Can you work these out from the drawing? Everything is in mm from the part's minimum corner. A direction names the side the tool comes from. Coordinates: 2 decimals unless noted, no trailing zeros. Loops run counter-clockwise (first coordinate to the right, second up) from the corner with the lowest first, then second, coordinate; pieces in that order, holes last.
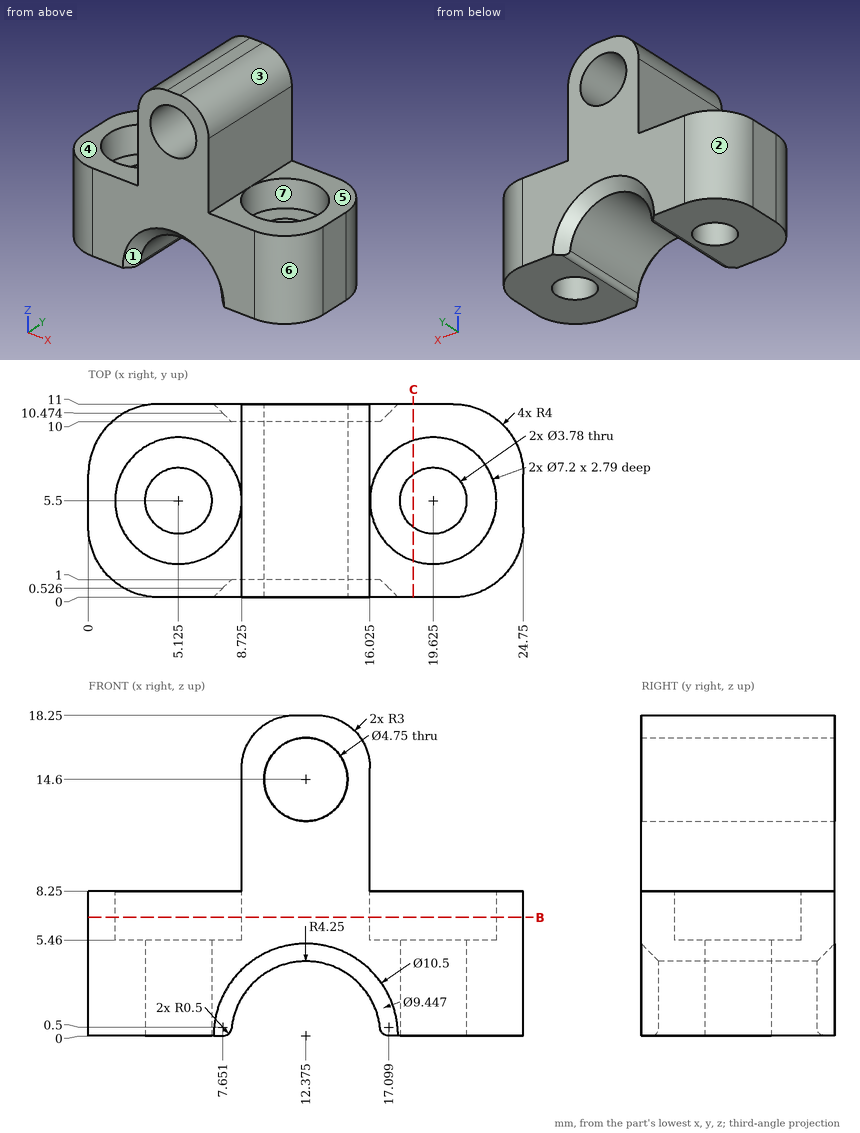
1. On a 3-axis mill with a long thin cutter (end or side, diameter ignored), from which of +Z, -Z, +X, -X, +Y, -Y can I reach the whole of each face in a straight line? I mean the marked faces 5, 6 and 7. Say none if no direction works.
2. We'd pull the mould along X, two halves only. Please class the marked faces 1, 2, 3 and 4: +X half, -X half, draft (parallel to the pull), parting line (faces both ways), or undercut.
3. For pin 1 (6 mm diameter, centred on x = 19.625, y = 5.5, fed in from +Z); pin 2 (1 mm diameter, centred on y = 5.5, z = 9, fed in from +X) (3 decimals); pin 3 (2 mm diameter, centred on y = 7, z = 10.5, fed in from -X) (3 decimals), each with a flat end and sliding along its axis, tell me the tip position at first contact or that it passes through.
4. I want a section at B-B (z = 6.75). Give the number of separate pieces and of enclosed holes in the cut face, then the cut area to 3 significant figures.
5. I want a section at C-C (x = 18.5). Please give me the cut outline in (y, z).
6. I need wall thicknesses on line 1 along Z through (x, y) = (7.5, 4.5); line 2 along Z through (x, y) = (23, 10.25); line 3 along Z through (x, y) = (14.5, 2) (1 decimal). Which ranges of each line are inside material? Lowest first, please.
Response values:
1. face 5: +Z, +X, +Y, -Y
1. face 6: +Z, -Z, +X, -Y
1. face 7: +Z
2. face 1: undercut
2. face 2: -X half
2. face 3: +X half
2. face 4: draft
3. pin 1: stops at z = 5.46
3. pin 2: stops at x = 16.025
3. pin 3: stops at x = 8.725
4. separate pieces: 1
4. enclosed holes: 2
4. area: 177 mm2
5. outline: (0, 0) - (3.98, 0) - (3.98, 5.46) - (2.08, 5.46) - (2.08, 8.25) - (0, 8.25) - close; (7.02, 0) - (11, 0) - (11, 8.25) - (8.92, 8.25) - (8.92, 5.46) - (7.02, 5.46) - close
6. line 1: z = 0 to 5.46
6. line 2: z = 0 to 8.25
6. line 3: z = 3.7 to 13.5, 15.7 to 17.9
